Autodesk Fusion 360 part; units mm, degrees
sketch "Sketch1" plane through (0, 0, 0) normal (0, 1, 0) x (1, 0, 0)
  circle A0 centre (0, 0) radius 12.5
  dimension "d1" = 25
extrude "Extrude1" add sketch "Sketch1" along normal blind 105
sketch "Sketch2" plane through (0, 105, 0) normal (0, 1, 0) x (-1, 0, 0)
  circle A0 centre (0, 0) radius 12.5
  line L0 (-5.25, -2.75) -> (5.25, -2.75)
  line L1 (5.25, -2.75) -> (5.25, 2.75)
  line L2 (5.25, 2.75) -> (-5.25, 2.75)
  line L3 (-5.25, 2.75) -> (-5.25, -2.75)
  line L4 (-5.25, -2.75) -> (5.25, 2.75) construction
  line L5 (5.25, -2.75) -> (-5.25, 2.75) construction
  dimension "d4" = 10.5
  dimension "d5" = 5.5
extrude "Extrude2" cut sketch "Sketch2" against normal blind 8 contours L0 L1 L2 L3
sketch "Sketch3" plane through (0, 0, 0) normal (0, -1, 0) x (1, 0, 0)
  circle A0 centre (0, 0) radius 12.5
extrude "Extrude3" cut sketch "Sketch2" along normal blind 8 from surface at -105 contours L0 L1 L2 L3
Input: part model. Units: mm. Frame: model coordinates. A direction names the side the tool comes from. Give positions to 0.01 mm unless a question says otherwise; leave off trailing zeros. Order: outer loops, then holes, each group sorted by start corner. A loop starts at its lowest first (then second) coordinate and runs counter-clockwise, first axis right, second up. Notation, with made-up numbers: (40, -22) - (44, -22) arc R11 cw to (44, -18) - close; hole circle Ø10 at (44, -30.75). An arc over 180 degrees is marked (long way). Put each result on its own line as item: value.
Item 1: Ray query, L1, parallel to Z at x = 0, y = 18; L2, parallel to Y at x = -4.75, z = 0; L3, parallel to Z at x = 10.75, y = 29. Return the intervals inside material, ascending. Write a range as from..to.
Found:
L1: z = -12.5..12.5
L2: y = 8..97
L3: z = -6.38..6.38
Item 2: Section query B-B, the plane x = -0.75. Return loops of the section in (y, z), then the cut area to 3 significant figures.
Found:
outline: (0, -12.48) - (105, -12.48) - (105, -2.75) - (97, -2.75) - (97, 2.75) - (105, 2.75) - (105, 12.48) - (0, 12.48) - (0, 2.75) - (8, 2.75) - (8, -2.75) - (0, -2.75) - close
area: 2,530 mm^2
Item 3: Access query for faces 5 (the flat face through (-5.25, 4, 0)), 6 (the flat face through (0, 105, -3)), 7 (the flat face through (0, 101, -2.75)). Directions: +Z, -Z, +X, -X, +Y, -Y. A direction counts if a zero-diameter tool reaches every point of the face in a straight line with its end or side. Return the directions, or none.
Found:
face 5: -Y
face 6: +Z, -Z, +X, -X, +Y
face 7: +Y
Item 4: Draft query along Z for faces 1 (the flat face through (0, 0, -3)), 2 (the cylindrical face through (11.923, 51.765, 3.755)), 3 (the flat face through (0, 101, 2.75)), 4 (the flat face through (5.25, 4, 0)). Return one class per face: +Z half, -Z half, draft (parallel to the pull), parting line (faces both ways), or undercut.
Found:
face 1: draft
face 2: parting line
face 3: undercut
face 4: undercut
Item 5: Section query A-A, the plane z = 0. Return loops of the section in (x, y), then the cut area to 3 significant figures.
Found:
outline: (-12.5, 0) - (-5.25, 0) - (-5.25, 8) - (5.25, 8) - (5.25, 0) - (12.5, 0) - (12.5, 105) - (5.25, 105) - (5.25, 97) - (-5.25, 97) - (-5.25, 105) - (-12.5, 105) - close
area: 2,460 mm^2
Item 6: Section query D-D, the plane x = 10. Return loops of the section in (y, z).
Found:
outline: (0, -7.5) - (105, -7.5) - (105, 7.5) - (0, 7.5) - close
Item 7: Section query C-C, the plane y = 82. Return loops of the section in (x, z), then the cut area to 3 significant figures.
Found:
outline: circle Ø25 at (0, 0)
area: 491 mm^2
Item 8: Contact query for flat-ended pins moving along their axis: pin 1 (2.5 mm diameter, centred on x = 1.5, y = 4, fed in from -Z); pin 2 (3 mm diameter, centred on y = 34.5, z = 3, fed in from +X); pin 3 (3 mm diameter, centred on y = 42, z = -8, fed in from -X). Output: stop coordinate, or through.
Found:
pin 1: stops at z = -12.5
pin 2: stops at x = 12.41
pin 3: stops at x = -10.68
